The listing builds one solid part. Answer for the finished solid, in the listing's coordinates (mm). A direction names the side the tool comes from. Coordinates: 2 decimals unless noted, no trailing zeros. Loops run counter-clockwise (first coordinate to the right, second up) from the corner with the lowest first, then second, coordinate; pieces in that order, holes last. Notation, with made-up numbers: M -28,55.25 L 4,55.25 A13 cw 4,62.25 Z; hole C 34.5,8 d4. An arc over 180 degrees is marked long. Answer as a JSON object with one key per item and string values. Group by question number.
1. A cutting plane is placed at D-D on z = -92. Give the vertices of the cut face in (x, y) (3 decimals).
2. Straight lines are drawn through the part: L1, parallel to X at y = -16.5, z = -11; L2, parallel to Y at x = 5.25, z = 0 (3 decimals); L3, parallel to Z at x = -40, y = 1. For each, find the intervals that lie inside material, in ascending order.
3. For faces 1 (the face through (25.4, 0, -305)), 2 (the face through (-10, 0, -308.521)), 3 (the face through (16, 0, -308.521)), determine the directions among +Z, -Z, +X, -X, +Y, -Y from which every point of the face is accessible in a straight line to the end or side of a thin tool.
4. A cutting plane is placed at C-C on x = 38. Give the vertices of the cut face in (y, z) (3 decimals).
5. A cutting plane is placed at A-A on x = -68. Give the vertices of the cut face in (y, z) (3 decimals), and give its area (3 significant figures).
6. Given pin 1 (6.5 mm diameter, centred on y = 1.5, z = -323.5, fed in from -X) (3 decimals); pin 2 (1.9 mm diameter, centred on y = 0.5, z = -304, fed in from +X); pin 3 (6 mm diameter, centred on y = 0, z = -87, fed in from -X), each flat-ended and moving along its own axis, determine where each tip first touches the part or whether it passes through.
7. Determine the mould class of faces 4 (the face through (2.899, 0.774, 18.547)), 5 (the face through (17, 3.175, -121)), 6 (the face through (3.219, 3.905, -0.867)), 7 (the face through (15.875, 0, -322)) for opening direction Y: released by +Y, released by -Y, zero draft, split by the parting line, or undercut.
from build123d import *

# Parameters (mm, degrees)
BOSS_EXTRUDE1_REACH     = 30.816
SKETCH2_R               = 4
BOSS_EXTRUDE4_DEPTH     = 6.35
CUT_EXTRUDE1_DEPTH      = 325.659613706
CUT_EXTRUDE1_DEPTH_BACK = 325.659613706
BOSS_EXTRUDE5_DEPTH     = 3.175
BOSS_EXTRUDE6_DEPTH     = 12.7


with BuildPart() as part:
    # Sketch1 → Revolve1 (revolve)
    with BuildSketch(Plane.XY, mode=Mode.PRIVATE) as revolve1_sk:
        Polygon((0, 4), (6.35, 4), (6.35, 19.875), (4.7625, 19.875), (3.175, 18.2875), (1.5875, 19.875), (0, 19.875), align=None)
    revolve(revolve1_sk.sketch.rotate(Axis((0, 0, 0), (1, 0, 0)), 90), axis=Axis((0, 0, 0), (1, 0, 0)))

    # Boss-Extrude1: up to this face of the body (flat: up to its plane)
    boss_extrude1_end = Plane(part.part.faces().sort_by_distance((0, 0, -19.312850109))[0])
    # Sketch2 → Boss-Extrude1 (add, up to the picked face)
    with BuildSketch(Plane(origin=(6.35, 0, 0), x_dir=(0, 0, -1), z_dir=(1, 0, 0)), mode=Mode.PRIVATE) as boss_extrude1_sk1:
        with BuildLine():
            Line((20.028068585, 3.175), (304.8, 3.175))
            Line((304.8, 3.175), (304.8, 0))
            Line((304.8, 0), (304.8, -3.175))
            Line((304.8, -3.175), (20.028068585, -3.175))
            ThreePointArc((20.028068585, -3.175), (18.498150057, -3.687452393), (17.585562562, -5.018032049))
            ThreePointArc((17.585562562, -5.018032049), (-18.2875, 0), (17.585562562, 5.018032049))
            ThreePointArc((17.585562562, 5.018032049), (18.498150057, 3.687452393), (20.028068585, 3.175))
        make_face()
        with Locations(Location((0, 0, 0), (0, 0, 180))):
            Circle(SKETCH2_R, mode=Mode.SUBTRACT)
    boss_extrude1_tool1 = split(extrude(boss_extrude1_sk1.sketch, amount=-BOSS_EXTRUDE1_REACH, mode=Mode.PRIVATE), bisect_by=boss_extrude1_end, keep=Keep.BOTH, mode=Mode.PRIVATE)
    add(boss_extrude1_tool1.solids().sort_by(Axis((6.35, 0, -104.167204), (-1, 0, 0)))[0])

    # Sketch6 → Boss-Extrude4 (add)
    with BuildSketch(Plane.XZ.offset(3.175)):
        with BuildLine():
            ThreePointArc((0, -114.352931374), (-91.58879889, -199.938292555), (-19.05, -302.170796126))
            ThreePointArc((-19.05, -302.170796126), (-9.590159419, -303.940747454), (0, -304.747068626))
            Line((0, -304.747068626), (0, -298.393285481))
            ThreePointArc((0, -298.393285481), (-85.725, -209.55), (0, -120.706714519))
            Line((0, -120.706714519), (0, -114.352931374))
        make_face()
        with BuildLine():
            ThreePointArc((98.425, -209.55), (71.640251223, -143.330124774), (6.35, -114.352931374))
            Line((6.35, -114.352931374), (6.35, -120.706714519))
            ThreePointArc((6.35, -120.706714519), (67.149477333, -147.820944848), (92.075, -209.55))
            ThreePointArc((92.075, -209.55), (67.149477333, -271.279055152), (6.35, -298.393285481))
            Line((6.35, -298.393285481), (6.35, -304.747068626))
            ThreePointArc((6.35, -304.747068626), (15.940159419, -303.940747454), (25.4, -302.170796126))
            ThreePointArc((25.4, -302.170796126), (77.973040583, -268.523007597), (98.425, -209.55))
        make_face()
        with BuildLine():
            ThreePointArc((0, -304.747068626), (-9.590159419, -303.940747454), (-19.05, -302.170796126))
            Line((-19.05, -302.170796126), (-19.05, -308.520796126))
            Line((-19.05, -308.520796126), (25.4, -308.520796126))
            Line((25.4, -308.520796126), (25.4, -302.170796126))
            ThreePointArc((25.4, -302.170796126), (15.940159419, -303.940747454), (6.35, -304.747068626))
            Line((6.35, -304.747068626), (6.35, -304.8))
            Line((6.35, -304.8), (3.175, -304.8))
            Line((3.175, -304.8), (0, -304.8))
            Line((0, -304.8), (0, -304.747068626))
        make_face()
    extrude(amount=-BOSS_EXTRUDE4_DEPTH)

    # Sketch6<4> → Cut-Extrude1 (cut, two sides: drawn at the far end of the back side and taken through both)
    with BuildSketch(Plane.XZ.offset(3.175).offset(-CUT_EXTRUDE1_DEPTH_BACK)):
        with BuildLine():
            ThreePointArc((0, -298.393285481), (1.58724675, -298.435820239), (3.175, -298.45))
            Line((3.175, -298.45), (3.175, -120.65))
            ThreePointArc((3.175, -120.65), (1.58724675, -120.664179761), (0, -120.706714519))
            Line((0, -120.706714519), (0, -298.393285481))
        make_face()
        with BuildLine():
            Line((3.175, -120.65), (3.175, -298.45))
            ThreePointArc((3.175, -298.45), (4.76275325, -298.435820239), (6.35, -298.393285481))
            Line((6.35, -298.393285481), (6.35, -120.706714519))
            ThreePointArc((6.35, -120.706714519), (4.76275325, -120.664179761), (3.175, -120.65))
        make_face()
    extrude(amount=CUT_EXTRUDE1_DEPTH + CUT_EXTRUDE1_DEPTH_BACK, mode=Mode.SUBTRACT)

    # Sketch8 → Boss-Extrude5 (add, symmetric)
    with BuildSketch(Plane.ZY.offset(-3.175)):
        with BuildLine():
            Line((-308.520796126, -3.175), (-308.520796126, 3.175))
            Line((-308.520796126, 3.175), (-321.183816784, 3.96869459))
            ThreePointArc((-321.183816784, 3.96869459), (-318.683458763, 2.645954285), (-317.683279744, 0))
            ThreePointArc((-317.683279744, 0), (-318.683458763, -2.645954285), (-321.183816784, -3.96869459))
            Line((-321.183816784, -3.96869459), (-308.520796126, -3.175))
        make_face()
    extrude(amount=BOSS_EXTRUDE5_DEPTH, both=True)

    # Sketch8<3> → Boss-Extrude6 (add, symmetric)
    with BuildSketch(Plane.ZY.offset(-3.175)):
        with BuildLine():
            ThreePointArc((-317.683279744, 0), (-318.683458763, 2.645954285), (-321.183816784, 3.96869459))
            Line((-321.183816784, 3.96869459), (-321.683279744, 4))
            ThreePointArc((-321.683279744, 4), (-325.683279744, 0), (-321.683279744, -4))
            Line((-321.683279744, -4), (-321.183816784, -3.96869459))
            ThreePointArc((-321.183816784, -3.96869459), (-318.683458763, -2.645954285), (-317.683279744, 0))
        make_face()
    extrude(amount=BOSS_EXTRUDE6_DEPTH, both=True)


solid = part.part
From the geometry:
{
 "1": {"outline": "M 0,-3.175 L 6.35,-3.175 L 6.35,3.175 L 0,3.175 Z"},
 "2": {"L1": "x = 0 to 1.63, 4.72 to 6.35", "L2": "y = -19.875 to -4, 4 to 19.875", "L3": "z = -294.45 to -287.26, -131.84 to -124.65"},
 "3": {"face 1": "-Z, +X, +Y, -Y", "face 2": "-X, +Y, -Y", "face 3": "+X, +Y, -Y"},
 "4": {"outline": "M -3.175,-298.205 L 3.175,-298.205 L 3.175,-291.345 L -3.175,-291.345 Z; M -3.175,-127.755 L 3.175,-127.755 L 3.175,-120.895 L -3.175,-120.895 Z"},
 "5": {"outline": "M -3.175,-272.848 L 3.175,-272.848 L 3.175,-262.817 L -3.175,-262.817 Z; M -3.175,-156.283 L 3.175,-156.283 L 3.175,-146.252 L -3.175,-146.252 Z", "area": "127 mm²"},
 "6": {"pin 1": "stops at x = -9.525", "pin 2": "stops at x = 25.4", "pin 3": "stops at x = 0"},
 "7": {"face 4": "split by the parting line", "face 5": "released by +Y", "face 6": "undercut", "face 7": "zero draft"}
}
